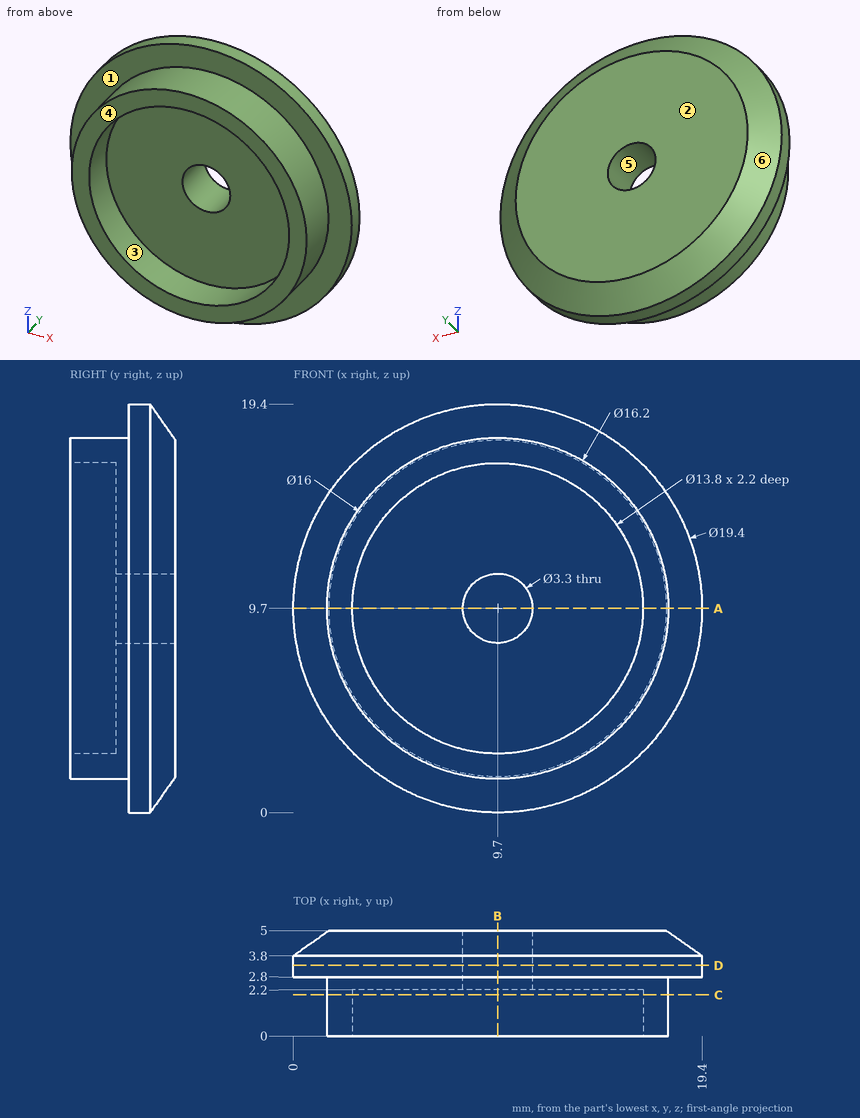
Design review of the part shown in the three views and the two pictorial views. Dimensions are in mm from the part's minimum x, y and z. A direction names the side the tool comes from. Give positions to 0.01 mm unless a question says otherwise; leave off trailing zeros. Loops run counter-clockwise (first coordinate to the right, second up) from the corner with the lowest first, then second, coordinate; pieces in that order, holes last. Notation, with made-up numbers: (-7.5, 47.25) -> (33.5, 47.25) arc R36 ccw to (33.5, 81.25) -> close; hole circle Ø5 at (-2.75, -22.75). An arc over 180 degrees is marked (long way). Answer as a JSON object with one key per item and string values. Group by question number.
Q1. Take a section at A-A (z = 9.7). Write out the cut boundary in (x, y).
Q2. Tool access review of the marked faces 1 and 2: name each direction out of +Z, -Z, +X, -X, +Y, -Y from which nothing blocks a thin tool from reaching the whole face with its end or side.
Q3. Insertion check: pin 1 (6 mm diameter, centred on x = 7.5, z = 7.5, fed in from -Y); pin 2 (2 mm diameter, centred on x = 4.5, y = 3.5, fed in from +Z); pin 3 (1 mm diameter, centred on x = 4.5, y = 3.5, fed in from +Z). Each pin has a flat end and moves straight along its axis. Give the tip position at first contact, or say it passes through.
Q4. Take a section at B-B (x = 9.7). Write out the cut boundary in (y, z).
Q5. Draft analysis for pull direction Z (two halves, no side actions). For the marked faces 3, 4, 5 and 6, state which applies: pulls with the +Z half, pulls with the -Z half, needs draft (parallel to the pull), parting line crosses it, or undercut.
Q6. Take a section at D-D (y = 3.35). Write out the cut boundary in (x, z), plus the area to 3 significant figures.
Q7. Take a section at C-C (y = 1.95). Write out the cut boundary in (x, z), plus the area to 3 significant figures.
Q8. Wall thickness on line 1 along Z through (x, y) = (9.7, 0.9); line 2 along X through (y, z) = (3.4, 9.7): over which ranges is each line inside the solid? List them lowest first.
Answer below:
{
 "1": {"outline": "(0, 2.8) -> (1.6, 2.8) -> (1.6, 0) -> (2.8, 0) -> (2.8, 2.2) -> (8.05, 2.2) -> (8.05, 5) -> (1.7, 5) -> (0, 3.8) -> close; (11.35, 2.2) -> (16.6, 2.2) -> (16.6, 0) -> (17.8, 0) -> (17.8, 2.8) -> (19.4, 2.8) -> (19.4, 3.8) -> (17.7, 5) -> (11.35, 5) -> close"},
 "2": {"face 1": "-Y", "face 2": "+Z, -Z, +X, -X, +Y"},
 "3": {"pin 1": "stops at y = 2.2", "pin 2": "stops at z = 18.44", "pin 3": "stops at z = 18.19"},
 "4": {"outline": "(0, 1.6) -> (2.8, 1.6) -> (2.8, 0) -> (3.8, 0) -> (5, 1.7) -> (5, 8.05) -> (2.2, 8.05) -> (2.2, 2.8) -> (0, 2.8) -> close; (0, 16.6) -> (2.2, 16.6) -> (2.2, 11.35) -> (5, 11.35) -> (5, 17.7) -> (3.8, 19.4) -> (2.8, 19.4) -> (2.8, 17.8) -> (0, 17.8) -> close"},
 "5": {"face 3": "undercut", "face 4": "needs draft", "face 5": "undercut", "face 6": "parting line crosses it"},
 "6": {"outline": "circle Ø19.4 at (9.7, 9.7); hole circle Ø3.3 at (9.7, 9.7)", "area": "287 mm2"},
 "7": {"outline": "circle Ø16.2 at (9.7, 9.7); hole circle Ø13.8 at (9.7, 9.7)", "area": "56.5 mm2"},
 "8": {"line 1": "z = 1.6 to 2.8, 16.6 to 17.8", "line 2": "x = 0 to 8.05, 11.35 to 19.4"}
}
